Read the model definition and answer for the solid it produces. Units are mm, in the model's axes. A direction names the side the tool comes from. Give positions to 0.01 mm unless a question says otherwise; leave off trailing zeros. Loops run counter-clockwise (first coordinate to the right, second up) from the corner with the lowest first, then second, coordinate; pieces in that order, holes last. Notation, with made-up numbers: M 60.25,76.25 L 79.25,76.25 A22 ccw 79.25,101.25 Z; hole C 0,84 d7. An arc over 180 degrees is marked long. Return JSON: item names as keys, results as strings. Group by question number.
```python
from build123d import *

# Parameters (mm, degrees)
F1_DEPTH  = 28
F2_W      = 27
F2_H      = 20
F3_DEPTH  = 27
F5_D      = 6.6
F7_D      = 6.6
F8_W      = 2.7
F8_H      = 8.1
F8_W_2    = 8.7
F9_DEPTH  = 2
F10_W     = 2.7
F10_H     = 8.1
F10_W_2   = 8.7
F11_DEPTH = 2
F12_SIZE  = 1
F13_W     = 2
F13_H     = 20
F14_DEPTH = 2.5


with BuildPart() as f1:
    # F0 (on Top) → F1 (new body)
    with BuildSketch(Plane.XY):
        Polygon((0, 32), (0, 0), (32, 0), (32, 5), (5, 32), align=None)
    extrude(amount=F1_DEPTH)

    # F2 (on face) → F3 (cut, through all)
    with BuildSketch(Plane.YZ.offset(32)):
        with Locations((18.5, 14)):
            Rectangle(F2_W, F2_H)
    extrude(amount=-F3_DEPTH, mode=Mode.SUBTRACT)

    # F5 (through all)
    with Locations(Plane.YZ.offset(5)):
        with Locations((19, 14)):
            Hole(F5_D / 2)

    # F7 (through all)
    with Locations(Plane(origin=(0, 5, 0), x_dir=(-1, 0, 0), z_dir=(0, 1, 0))):
        with Locations((-19, 14)):
            Hole(F7_D / 2)

    # F8 (on face) → F9 (join)
    with BuildSketch(Plane.XZ):
        with Locations((27.65, 14)):
            Rectangle(F8_W, F8_H)
        with Locations((7.35, 14)):
            Rectangle(F8_W_2, F8_H)
    extrude(amount=F9_DEPTH)

    # F10 (on face) → F11 (join)
    with BuildSketch(Plane(origin=(0, 0, 0), x_dir=(0, -1, 0), z_dir=(-1, 0, 0))):
        with Locations((-27.65, 14)):
            Rectangle(F10_W, F10_H)
        with Locations((-7.35, 14)):
            Rectangle(F10_W_2, F10_H)
    extrude(amount=F11_DEPTH)

    # F12
    f12_edges = [f1.edges().sort_by_distance(p)[0] for p in [
        (0, 32, 14),
        (-2, 29, 14),
        (-2, 26.3, 14),
        (-2, 11.7, 14),
        (-2, 3, 14),
        (0, 0, 14),
        (3, -2, 14),
        (11.7, -2, 14),
        (26.3, -2, 14),
        (29, -2, 14),
        (32, 0, 14),
    ]]
    chamfer(f12_edges, length=F12_SIZE)

    # F13 (on face) → F14 (join)
    with BuildSketch(Plane(origin=(18.5, 18.5, 0), x_dir=(-0.7071067812, 0.7071067812, 0), z_dir=(0.7071067812, 0.7071067812, 0))):
        with Locations((-18.091883092, 14)):
            Rectangle(F13_W, F13_H)
        with Locations((18.091883092, 14)):
            Rectangle(F13_W, F13_H)
    extrude(amount=-F14_DEPTH)


solid = f1.part
```
1. Find section B-B (x = 10). Write down the section's boundary in (y, z).
2. Find section D-D (y = 7.5). Write down the section's boundary in (x, z).
3. Flat-ended cylindrical pins translate along their axes: P1, Ø0.6, axis at x = -0.5, y = 7, coming from the -Z side; P2, Ø0.5, axis at x = -0.5, z = 13, coming from the +Y side; P3, Ø0.8, axis at x = -0.5, z = 15.5, coming from the -Y side; P4, Ø7.5, axis at x = 12, y = 15, coming from the -Z side. Find the tip coordinate at first contact, or state that the pin passes through.
4. The mould has two halves that part along X. Classify faces 5 (the flat face through (11.2, -1.5, 13.9)), 6 (the flat face through (12, 13, 0)), 7 (the flat face through (-1.5, 26.8, 13.9)), 8 (the cylindrical face through (18.28, 2.47, 10.78)): +X half, -X half, draft (parallel to the pull), parting line (faces both ways), or undercut.
5. For faces 1 (the flat face through (-0.5, 11.7, 13.9)), 2 (the flat face through (7, -1, 18.05)), 3 (the flat face through (-0.5, 29, 13.9)), 4 (the flat face through (5, 14, 14)), determine the directions among +Z, -Z, +X, -X, +Y, -Y from which every point of the face is accessible in a straight line to the end or side of a thin tool.
6. Find section A-A (y = 19). Write down the section's boundary in (x, z), and give its area (3 significant figures).
7. Straight lines are drawn through the part: line 1 along Z through (x, y) = (1.75, 19); line 2 along Z through (x, y) = (6, 21.5); line 3 along X through (y, z) = (14.5, 8.25). For each, find the intervals that lie inside material, in ascending order.
Result:
{
 "1": {"outline": "M -2,9.95 L 0,9.95 L 0,0 L 27,0 L 27,4 L 5,4 L 5,24 L 27,24 L 27,28 L 0,28 L 0,18.05 L -2,18.05 Z"},
 "2": {"outline": "M -2,9.95 L 0,9.95 L 0,0 L 29.5,0 L 29.5,4 L 5,4 L 5,24 L 29.5,24 L 29.5,28 L 0,28 L 0,18.05 L -2,18.05 Z"},
 "3": {"P1": "stops at z = 9.95", "P2": "stops at y = 29", "P3": "stops at y = 3", "P4": "stops at z = 0"},
 "4": {"face 5": "undercut", "face 6": "draft", "face 7": "-X half", "face 8": "undercut"},
 "5": {"face 1": "+Z, -Z, -X", "face 2": "+Z, +X, -X, -Y", "face 3": "+Z, -Z, -X, +Y", "face 4": "none"},
 "6": {"outline": "M 0,0 L 18,0 L 18,4 L 5,4 L 5,10.7 L 0,10.7 Z; M 0,17.3 L 5,17.3 L 5,24 L 18,24 L 18,28 L 0,28 Z", "area": "211 mm2"},
 "7": {"line 1": "z = 0 to 10.7, 17.3 to 28", "line 2": "z = 0 to 4, 24 to 28", "line 3": "x = 0 to 5"}
}
